Job drawing, mm, ordinate dimensions from the low corner. One solid piece. Round coordinates to 2 decimals unless told otherwise and drop trailing zeros. Loops run counter-clockwise (first coordinate to the right, second up) from the corner with the lowest first, then second, coordinate; pieces in that order, holes last.
1) Band-saw the part on B-B, the plane x = 5. Write the cut outline in (y, z), then the cut area to 3 significant figures.
2) Band-saw the part on A-A, the plane y = 15. Write the cut outline in (x, z), then the cut area to 3 significant figures.
3) Band-saw the part on C-C, the plane z = 4.5. Write the cut outline in (x, y).
4) Drop flat-ended pins along their axis: P1, Ø5.5, axis at x = 35, y = 34, coming from the -Z side; P2, Ø0.5, axis at x = 34.5, z = 1, coming from the +Y side; P3, Ø0.5, axis at x = 34.5, z = 0.5, coming from the -Y side. Give the stop position or say it passes through.
5) Probe line 1 (Y direction, x = 35, z = 3.4); line 2 (Y direction, x = 20, z = 2.8); line 3 (X direction, y = 87, z = 2.5). List the from-to ranges inside material, lowest first.
6) Band-saw the part on D-D, the plane x = 19.5. Write the cut outline in (y, z).
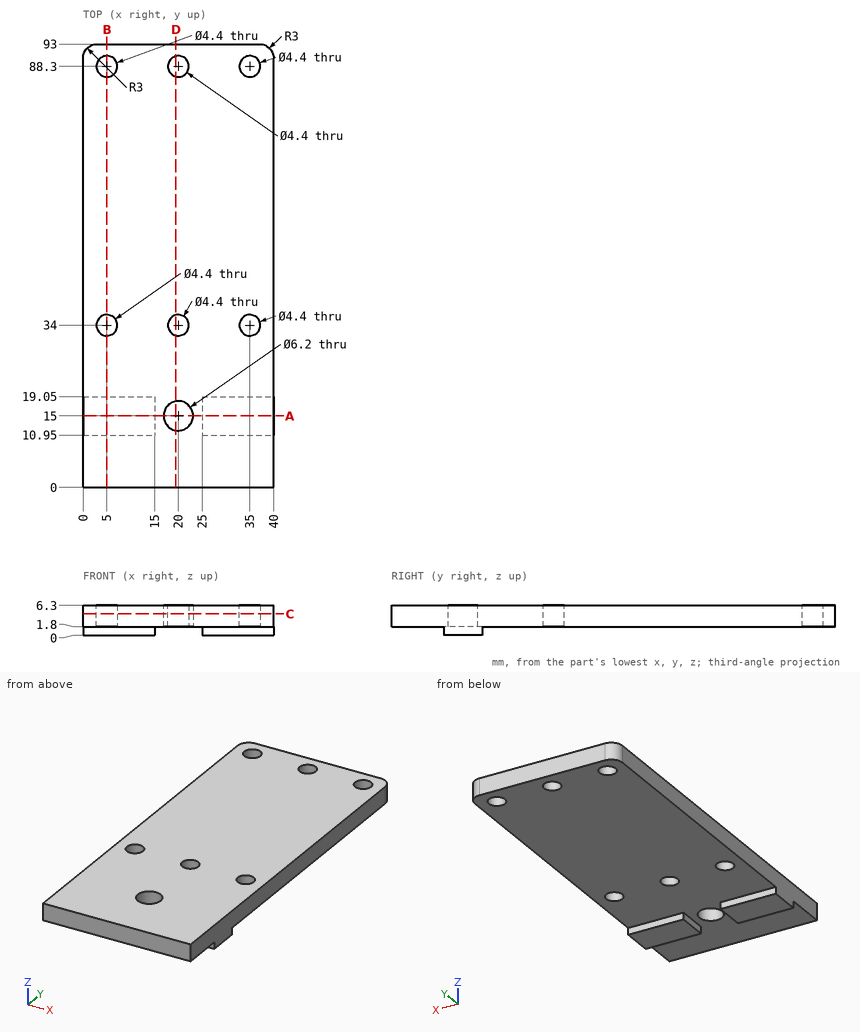
Reported:
1. outline: (0, 1.8) - (10.95, 1.8) - (10.95, 0) - (19.05, 0) - (19.05, 1.8) - (31.8, 1.8) - (31.8, 6.3) - (0, 6.3) - close; (36.2, 1.8) - (86.1, 1.8) - (86.1, 6.3) - (36.2, 6.3) - close; (90.5, 1.8) - (93, 1.8) - (93, 6.3) - (90.5, 6.3) - close
1. area: 393 mm2
2. outline: (0, 0) - (15, 0) - (15, 1.8) - (16.9, 1.8) - (16.9, 6.3) - (0, 6.3) - close; (23.1, 1.8) - (25, 1.8) - (25, 0) - (40, 0) - (40, 6.3) - (23.1, 6.3) - close
2. area: 206 mm2
3. outline: (0, 0) - (40, 0) - (40, 90) arc R3 ccw to (37, 93) - (3, 93) arc R3 ccw to (0, 90) - close; hole circle Ø4.4 at (5, 34); hole circle Ø4.4 at (5, 88.3); hole circle Ø6.2 at (20, 15); hole circle Ø4.4 at (20, 34); hole circle Ø4.4 at (20, 88.3); hole circle Ø4.4 at (35, 34); hole circle Ø4.4 at (35, 88.3)
4. P1: stops at z = 1.8
4. P2: stops at y = 19.05
4. P3: stops at y = 10.95
5. line 1: y = 0 to 31.8, 36.2 to 86.1, 90.5 to 93
5. line 2: y = 0 to 11.9, 18.1 to 31.8, 36.2 to 86.1, 90.5 to 93
5. line 3: x = 0 to 3.23, 6.77 to 18.23, 21.77 to 33.23, 36.77 to 40
6. outline: (0, 1.8) - (11.94, 1.8) - (11.94, 6.3) - (0, 6.3) - close; (18.06, 1.8) - (31.86, 1.8) - (31.86, 6.3) - (18.06, 6.3) - close; (36.14, 1.8) - (86.16, 1.8) - (86.16, 6.3) - (36.14, 6.3) - close; (90.44, 1.8) - (93, 1.8) - (93, 6.3) - (90.44, 6.3) - close
